Geometry check sheet. Reference: the model listing, model coordinates, mm. Face numbers are marked on the shaded views. A direction names the side the tool comes from. Give positions to 0.01 mm unless a question says otherwise; leave off trailing zeros. Loops run counter-clockwise (first coordinate to the right, second up) from the corner with the lowest first, then second, coordinate; pieces in that order, holes last. Notation, with made-up numbers: (30.5, -6) - (49.5, -6) arc R24 ccw to (49.5, 30) - close; hole circle Ø6 at (-23.5, 36.5). An arc over 180 degrees is marked (long way). Use a Markdown table: item, result. Add a question column.
1. Set-up check for the marked faces 1, 2 and 3: record each of +Z, -Z, +X, -X, +Y, -Y from which the full face is reachable in a straight line by a thin tool's end or side.
2. Draft check along Z on the marked faces 4, 5 and 6. Enter one of: pulls with the +Z half, pulls with the -Z half, needs draft (parallel to the pull), parting line crosses it, or undercut.
3. Material ranges on L1, parallel to Z at x = 8, y = 3; L2, parallel to Z at x = -5.5, y = -1.5; L3, parallel to X at y = -1.75, z = 9, recorded low to high.
4. Depth check by flat-ended pin: P1, Ø5.5, axis at x = -2, z = 1, coming from the -Y side; P2, Ø7, axis at x = 5.5, y = 4, coming from the -Z side; P3, Ø6, axis at y = -3.5, z = 18, coming from the +X side; P4, Ø1.5, axis at x = 7.5, y = -3, coming from the -Z side. Enter the tip coordinate at first touch or a pass-through.
5. Cross-section at B-B on z = -6. Enter the section's corners in (x, y), and give its area (3 significant figures).
6. Cross-section at C-C on y = 6.25. Enter the section's corners in (x, z), and give its area (3 significant figures).
7. Cross-section at A-A on x = -2. Enter the section's corners in (y, z).
8. Cross-section at D-D on x = -16. Enter the section's corners in (y, z), and give its area (3 significant figures).
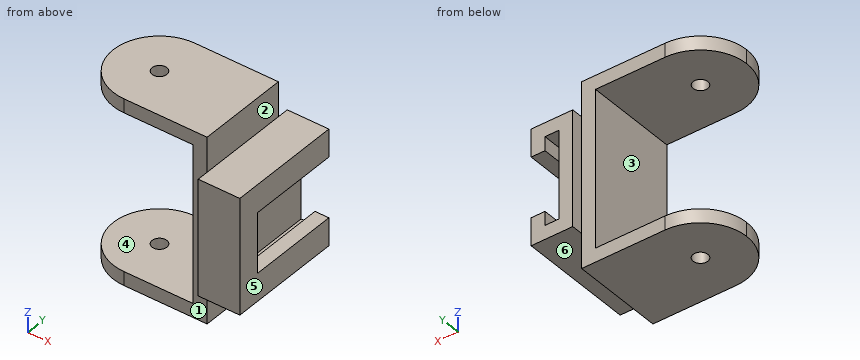
from build123d import *

# Parameters (mm, degrees)
ESQUISSE1_W             = 40
ESQUISSE1_H             = 20
BOSS_EXTRU_1_DEPTH      = 3
ESQUISSE2_W             = 3
ESQUISSE2_H             = 20
BOSS_EXTRU_2_DEPTH      = 25
ENL_V_MAT_EXTRU_1_DEPTH = 48
ESQUISSE4_R             = 1.6
ENL_V_MAT_EXTRU_2_DEPTH = 48
ESQUISSE5_W             = 25
ESQUISSE5_H             = 25
BOSS_EXTRU_3_DEPTH      = 9
ESQUISSE6_W             = 3
ESQUISSE6_H             = 19
ENL_V_MAT_EXTRU_4_DEPTH = 23
ESQUISSE8_W             = 13
ESQUISSE8_H             = 20
ENL_V_MAT_EXTRU_5_DEPTH = 3


with BuildPart() as part:
    # Esquisse1 → Boss.-Extru.1 (new body)
    with BuildSketch(Plane(origin=(0, 0, 0), x_dir=(0, 0, -1), z_dir=(1, 0, 0))):
        Rectangle(ESQUISSE1_W, ESQUISSE1_H)
    extrude(amount=BOSS_EXTRU_1_DEPTH)

    # Esquisse2 → Boss.-Extru.2 (add)
    with BuildSketch(Plane.ZY):
        with Locations((-18.5, 0)):
            Rectangle(ESQUISSE2_W, ESQUISSE2_H)
        with Locations((18.5, 0)):
            Rectangle(ESQUISSE2_W, ESQUISSE2_H)
    extrude(amount=BOSS_EXTRU_2_DEPTH)

    # Esquisse3 → Enlèv. mat.-Extru.1 (cut)
    with BuildSketch(Plane.XY.offset(20)):
        with BuildLine():
            ThreePointArc((-25, 2.7e-08), (-22.071067802, 7.071067821), (-15, 10))
            Line((-15, 10), (-25, 10))
            Line((-25, 10), (-25, 2.7e-08))
        make_face()
        with BuildLine():
            ThreePointArc((-15, -10), (-22.071067821, -7.071067802), (-25, 2.7e-08))
            Line((-25, 2.7e-08), (-25, -10))
            Line((-25, -10), (-15, -10))
        make_face()
    extrude(amount=-ENL_V_MAT_EXTRU_1_DEPTH, mode=Mode.SUBTRACT)

    # Esquisse4 → Enlèv. mat.-Extru.2 (cut)
    with BuildSketch(Plane.XY.offset(20)):
        with Locations((-15, 0)):
            Circle(ESQUISSE4_R)
    extrude(amount=-ENL_V_MAT_EXTRU_2_DEPTH, mode=Mode.SUBTRACT)

    # Esquisse5 → Boss.-Extru.3 (add)
    with BuildSketch(Plane(origin=(3, 0, 0), x_dir=(0, 0, -1), z_dir=(1, 0, 0))):
        Rectangle(ESQUISSE5_W, ESQUISSE5_H)
    extrude(amount=BOSS_EXTRU_3_DEPTH)

    # Esquisse6 → Enlèv. mat.-Extru.4 (cut)
    with BuildSketch(Plane(origin=(0, 12.5, 0), x_dir=(1, 0, 0), z_dir=(0, 1, 0))):
        with Locations((7.5, 0)):
            Rectangle(ESQUISSE6_W, ESQUISSE6_H)
    extrude(amount=-ENL_V_MAT_EXTRU_4_DEPTH, mode=Mode.SUBTRACT)

    # Esquisse8 → Enlèv. mat.-Extru.5 (cut)
    with BuildSketch(Plane(origin=(12, 0, 0), x_dir=(0, 0, -1), z_dir=(1, 0, 0))):
        with Locations((0, 2.5)):
            Rectangle(ESQUISSE8_W, ESQUISSE8_H)
    extrude(amount=-ENL_V_MAT_EXTRU_5_DEPTH, mode=Mode.SUBTRACT)


solid = part.part
Values found:
| question | item | result |
|---|---|---|
| 1 | face 1 | +Z, -Z, -X, -Y |
| 1 | face 2 | +Z, +X, +Y, -Y |
| 1 | face 3 | -X, +Y, -Y |
| 2 | face 4 | undercut |
| 2 | face 5 | needs draft |
| 2 | face 6 | pulls with the -Z half |
| 3 | L1 | z = -12.5 to -9.5, 9.5 to 12.5 |
| 3 | L2 | z = -20 to -17, 17 to 20 |
| 3 | L3 | x = 0 to 6, 9 to 12 |
| 4 | P1 | stops at y = -10 |
| 4 | P2 | stops at z = -20 |
| 4 | P3 | stops at x = 3 |
| 4 | P4 | stops at z = -12.5 |
| 5 | outline | (0, -10) - (3, -10) - (3, -12.5) - (12, -12.5) - (12, -7.5) - (9, -7.5) - (9, -10.5) - (6, -10.5) - (6, 12.5) - (3, 12.5) - (3, 10) - (0, 10) - close |
| 5 | area | 156 mm2 |
| 6 | outline | (-22.81, -20) - (3, -20) - (3, -12.5) - (12, -12.5) - (12, -6.5) - (9, -6.5) - (9, -9.5) - (6, -9.5) - (6, 9.5) - (9, 9.5) - (9, 6.5) - (12, 6.5) - (12, 12.5) - (3, 12.5) - (3, 20) - (-22.81, 20) - (-22.81, 17) - (0, 17) - (0, -17) - (-22.81, -17) - close |
| 6 | area | 386 mm2 |
| 7 | outline | (-10, -20) - (10, -20) - (10, -17) - (-10, -17) - close; (-10, 17) - (10, 17) - (10, 20) - (-10, 20) - close |
| 8 | outline | (-9.95, -20) - (-1.25, -20) - (-1.25, -17) - (-9.95, -17) - close; (-9.95, 17) - (-1.25, 17) - (-1.25, 20) - (-9.95, 20) - close; (1.25, -20) - (9.95, -20) - (9.95, -17) - (1.25, -17) - close; (1.25, 17) - (9.95, 17) - (9.95, 20) - (1.25, 20) - close |
| 8 | area | 104 mm2 |
